```python
from build123d import *

# Parameters (mm, degrees)
SKETCH_1_W           = 40
SKETCH_1_H           = 20
EXTRUDE_1_DEPTH      = 27.7
SKETCH_2_W           = 56
SKETCH_2_H           = 20
SKETCH_2_R           = 2
EXTRUDE_2_DEPTH      = 2.7
SKETCH_5_W           = 40
SKETCH_5_H           = 20
EXTRUDE_3_DEPTH      = 40
SKETCH_6_R           = 3
EXTRUDE_4_DEPTH      = 4.5
EXTRUDE_5_DEPTH      = 0.5
EXTRUDE_5_DEPTH_BACK = 1.5
SKETCH_7_R           = 10
SKETCH_8_R           = 1.5
CUT_EXTRUDE_4_DEPTH  = 2


with BuildPart() as part:
    # 草图1 → 凸台-拉伸1 (new body)
    with BuildSketch(Plane.XY):
        with Locations((-20, 10)):
            Rectangle(SKETCH_1_W, SKETCH_1_H)
    extrude(amount=EXTRUDE_1_DEPTH)

    # 草图2 → 凸台-拉伸2 (add)
    with BuildSketch(Plane.XY.offset(27.7)):
        with Locations((-20, 10)):
            Rectangle(SKETCH_2_W, SKETCH_2_H)
        with Locations(Location((-44.5, 15, 0), (0, 0, 180))):
            Circle(SKETCH_2_R, mode=Mode.SUBTRACT)
        with Locations(Location((-44.5, 5, 0), (0, 0, 180))):
            Circle(SKETCH_2_R, mode=Mode.SUBTRACT)
        with Locations(Location((4.5, 15, 0), (0, 0, 180))):
            Circle(SKETCH_2_R, mode=Mode.SUBTRACT)
        with Locations(Location((4.5, 5, 0), (0, 0, 180))):
            Circle(SKETCH_2_R, mode=Mode.SUBTRACT)
    extrude(amount=EXTRUDE_2_DEPTH)

    # 草图5 → 凸台-拉伸3 (add)
    with BuildSketch(Plane(origin=(0, 0, 0), x_dir=(-1, 0, 0), z_dir=(0, 0, -1))):
        with Locations((20, 10)):
            Rectangle(SKETCH_5_W, SKETCH_5_H)
    extrude(amount=-EXTRUDE_3_DEPTH)

    # 草图6 → 凸台-拉伸4 (add)
    with BuildSketch(Plane.XY.offset(40)):
        with Locations(Location((-10, 10, 0), (0, 0, 180))):
            Circle(SKETCH_6_R)
    extrude(amount=EXTRUDE_4_DEPTH)

    # 草图7 → 凸台-拉伸5 (add, two sides: drawn at the far end of the back side and taken through both)
    with BuildSketch(Plane.XY.offset(44.5).offset(-EXTRUDE_5_DEPTH_BACK)):
        with Locations((-10, 10)):
            Circle(SKETCH_7_R)
    extrude(amount=EXTRUDE_5_DEPTH + EXTRUDE_5_DEPTH_BACK)

    # 草图8 → 切除-拉伸4 (cut)
    with BuildSketch(Plane.XY.offset(45)):
        with Locations((-10, 10)):
            Circle(SKETCH_8_R)
        with Locations((-3, 10)):
            Circle(SKETCH_8_R)
        with Locations((-10, 17)):
            Circle(SKETCH_8_R)
        with Locations((-10, 3)):
            Circle(SKETCH_8_R)
        with Locations((-17, 10)):
            Circle(SKETCH_8_R)
    extrude(amount=-CUT_EXTRUDE_4_DEPTH, mode=Mode.SUBTRACT)


solid = part.part
```
Part model, mm, in its own coordinate system. A direction names the side the tool comes from. Coordinates: 2 decimals unless noted, no trailing zeros. Write each loop counter-clockwise with the first axis right and the second up, starting at its lowest first coordinate (ties: lowest second). Pieces come first, ordered by that corner, then holes.
Item 1: Slice it at A-A (y = 13.75). Write the cut outline in (x, z), and give its area (3 significant figures).
Item 2: Pin check, flat tips, straight feed: pin 1 (4 mm diameter, centred on x = 0.5, y = 11, fed in from -Z); pin 2 (2.5 mm diameter, centred on x = -44.5, y = 15, fed in from +Z); pin 3 (3 mm diameter, centred on x = -24, y = 6.5, fed in from +Z); pin 4 (7.5 mm diameter, centred on y = 9.5, z = 35, fed in from -X). Stop position of each tip, or through.
Item 3: Probe line 1 (X direction, y = 5, z = 28); line 2 (Z direction, x = -6, y = 12); line 3 (X direction, y = 4.75, z = 23). List the from-to ranges inside material, lowest first.
Item 4: Which spindle directions (+Z, -Z, +X, -X, +Y, -Y) get a long thin tool onto all of the face, cutting with end or side? Do faces 1 (the face through (-11.2, 2.1, 44)), 2 (the face through (-44, 10, 27.7)), 3 (the face through (-7.9, 12.4, 43)). Say none if no direction does.
Item 5: Slice it at B-B (y = 10). Count the separate pieces of the cut face and the enclosed holes in it, and give its area (3 significant figures).
Item 6: Slice it at C-C (x = -17). Write the cut outline in (y, z), and give its area (3 significant figures).
Item 7: Slice it at D-D (z = 7). Write the cut outline in (x, y).
Item 8: Mould opens along Z. For faces 4 (the face through (-8, 10, 45)), 5 (the face through (-12.17, 0.24, 43.99)), 6 (the face through (-20, 10, 40)), 7 (the face through (4, 10, 27.7)) say: released by +Z, released by -Z, zero draft, split by the parting line, or undercut.
Results found:
1. outline: (-48, 27.7) - (-46.06, 27.7) - (-46.06, 30.4) - (-48, 30.4) - close; (-42.94, 27.7) - (-40, 27.7) - (-40, 0) - (0, 0) - (0, 27.7) - (2.94, 27.7) - (2.94, 30.4) - (0, 30.4) - (0, 40) - (-40, 40) - (-40, 30.4) - (-42.94, 30.4) - close; (-19.27, 43) - (-0.73, 43) - (-0.73, 45) - (-19.27, 45) - close; (6.06, 27.7) - (8, 27.7) - (8, 30.4) - (6.06, 30.4) - close
1. area: 1,660 mm2
2. pin 1: stops at z = 0
2. pin 2: passes through
2. pin 3: stops at z = 40
2. pin 4: stops at x = -40
3. line 1: x = -48 to -46.5, -42.5 to 2.5, 6.5 to 8
3. line 2: z = 0 to 40, 43 to 45
3. line 3: x = -40 to 0
4. face 1: +Z
4. face 2: -Z, -X, +Y, -Y
4. face 3: none
5. separate pieces: 3
5. enclosed holes: 0
5. area: 1,680 mm2
6. outline: (0, 0) - (20, 0) - (20, 40) - (0, 40) - close; (2.86, 43) - (8.5, 43) - (8.5, 45) - (2.86, 45) - close; (11.5, 43) - (17.14, 43) - (17.14, 45) - (11.5, 45) - close
6. area: 823 mm2
7. outline: (-40, 0) - (0, 0) - (0, 20) - (-40, 20) - close
8. face 4: released by +Z
8. face 5: zero draft
8. face 6: undercut
8. face 7: released by -Z
